Read the model definition and answer for the solid it produces. Units are mm, in the model's axes. A direction names the side the tool comes from. Give positions to 0.01 mm unless a question says otherwise; leave off trailing zeros. Write each loop counter-clockwise with the first axis right and the second up, starting at its lowest first coordinate (ties: lowest second). Pieces come first, ordered by that corner, then holes. Notation, with made-up numbers: (24.25, 14) - (76.25, 14) arc R27 ccw to (76.25, 34) - close; hole circle Ø9 at (-9, 58.5). An arc over 180 degrees is marked (long way). Use CSV: the item, a comma, the result in double quotes. Start each with the question number.
from build123d import *

# Parameters (mm, degrees)
F1_DEPTH = 50.8
F2_R     = 6.35
F3_R     = 1.016


# Not quite as in the source:
# - a fillet or chamfer that OpenCascade refuses, or shapes differently, is made with other operations: its cross-section is extruded or revolved along the edge and cut away or added


with BuildPart() as f1:
    # F0 (on Top) → F1 (new body)
    with BuildSketch(Plane.XY):
        with BuildLine():
            ThreePointArc((-2.6150272293, 15.9155984364), (-1.9815871124, 16.0068095983), (-1.3450272293, 16.07282))
            Line((-1.3450272293, 16.07282), (-1.3450272293, 21.15282))
            Line((-1.3450272293, 21.15282), (-2.6150272293, 21.15282))
            Line((-2.6150272293, 21.15282), (-2.6150272293, 15.9155984364))
        make_face()
        with BuildLine():
            Line((1.3450272293, 21.15282), (1.3450272293, 16.07282))
            ThreePointArc((1.3450272293, 16.07282), (1.9815871124, 16.0068095983), (2.6150272293, 15.9155984364))
            Line((2.6150272293, 15.9155984364), (2.6150272293, 21.15282))
            Line((2.6150272293, 21.15282), (1.3450272293, 21.15282))
        make_face()
        with BuildLine():
            ThreePointArc((0, 15.621), (11.0457150289, 11.0457150289), (15.621, 0))
            ThreePointArc((15.621, 0), (15.0887273325, -4.0430123035), (13.5281828325, -7.8105))
            Line((13.5281828325, -7.8105), (13.9681237376, -8.0645))
            ThreePointArc((13.9681237376, -8.0645), (14.2925051104, -7.4745527405), (14.5919840451, -6.8715822506))
            ThreePointArc((14.5919840451, -6.8715822506), (14.8530973018, -6.28730002), (15.090826177, -5.693119206))
            ThreePointArc((15.090826177, -5.693119206), (15.867333998, -2.8935018222), (16.129, 0))
            ThreePointArc((16.129, 0), (12.2947634215, 10.439513083), (2.6150272293, 15.9155984364))
            ThreePointArc((2.6150272293, 15.9155984364), (1.9815871124, 16.0068095983), (1.3450272293, 16.07282))
            ThreePointArc((1.3450272293, 16.07282), (0.6731, 16.1149488795), (0, 16.129))
            Line((0, 16.129), (0, 15.621))
        make_face()
        with BuildLine():
            ThreePointArc((15.090826177, -5.693119206), (14.8530973018, -6.28730002), (14.5919840451, -6.8715822506))
            Line((14.5919840451, -6.8715822506), (18.9913930963, -9.4115822506))
            Line((18.9913930963, -9.4115822506), (19.6263930963, -8.3117299878))
            Line((19.6263930963, -8.3117299878), (15.090826177, -5.693119206))
        make_face()
        with BuildLine():
            Line((17.646365867, -11.7412377494), (13.2469568158, -9.2012377494))
            ThreePointArc((13.2469568158, -9.2012377494), (12.8744329677, -9.7156377434), (12.4819459699, -10.2149726287))
            Line((12.4819459699, -10.2149726287), (16.8813550211, -12.7549726287))
            Line((16.8813550211, -12.7549726287), (17.646365867, -11.7412377494))
        make_face()
        with BuildLine():
            Line((13.9681237376, -8.0645), (13.5281828325, -7.8105))
            ThreePointArc((13.5281828325, -7.8105), (0, -15.621), (-13.5281828325, -7.8105))
            Line((-13.5281828325, -7.8105), (-13.9681237376, -8.0645))
            ThreePointArc((-13.9681237376, -8.0645), (-13.6194051104, -8.6403961391), (-13.2469568158, -9.2012377494))
            ThreePointArc((-13.2469568158, -9.2012377494), (-12.8744329677, -9.7156377434), (-12.4819459699, -10.2149726287))
            ThreePointArc((-12.4819459699, -10.2149726287), (0, -16.129), (12.4819459699, -10.2149726287))
            ThreePointArc((12.4819459699, -10.2149726287), (12.8744329677, -9.7156377434), (13.2469568158, -9.2012377494))
            ThreePointArc((13.2469568158, -9.2012377494), (13.6194051104, -8.6403961391), (13.9681237376, -8.0645))
        make_face()
        with BuildLine():
            ThreePointArc((-12.4819459699, -10.2149726287), (-12.8744329677, -9.7156377434), (-13.2469568158, -9.2012377494))
            Line((-13.2469568158, -9.2012377494), (-17.646365867, -11.7412377494))
            Line((-17.646365867, -11.7412377494), (-16.8813550211, -12.7549726287))
            Line((-16.8813550211, -12.7549726287), (-12.4819459699, -10.2149726287))
        make_face()
        with BuildLine():
            ThreePointArc((-13.5281828325, -7.8105), (-13.5281828325, 7.8105), (0, 15.621))
            Line((0, 15.621), (0, 16.129))
            ThreePointArc((0, 16.129), (-0.6731, 16.1149488795), (-1.3450272293, 16.07282))
            ThreePointArc((-1.3450272293, 16.07282), (-1.9815871124, 16.0068095983), (-2.6150272293, 15.9155984364))
            ThreePointArc((-2.6150272293, 15.9155984364), (-13.970548685, 8.0602984088), (-15.0873987804, -5.7021959842))
            ThreePointArc((-15.0873987804, -5.7021959842), (-14.8512055836, -6.2917671377), (-14.5919840451, -6.8715822506))
            ThreePointArc((-14.5919840451, -6.8715822506), (-14.2925051104, -7.4745527405), (-13.9681237376, -8.0645))
            Line((-13.9681237376, -8.0645), (-13.5281828325, -7.8105))
        make_face()
        with BuildLine():
            Line((-18.9913930963, -9.4115822506), (-14.5919840451, -6.8715822506))
            ThreePointArc((-14.5919840451, -6.8715822506), (-14.8512055836, -6.2917671377), (-15.0873987804, -5.7021959842))
            Line((-15.0873987804, -5.7021959842), (-19.4868078316, -8.2421959842))
            Line((-19.4868078316, -8.2421959842), (-18.9913930963, -9.4115822506))
        make_face()
    extrude(amount=F1_DEPTH)

    # F2
    f2_edges = [f1.edges().sort_by_distance(p)[0] for p in [
        (2.615027, 15.915598, 25.4),
        (15.090826, -5.693119, 25.4),
        (12.481946, -10.214973, 25.4),
        (-12.481946, -10.214973, 25.4),
        (-15.087399, -5.702196, 25.4),
        (-2.615027, 15.915598, 25.4),
    ]]
    fillet(f2_edges, radius=F2_R)

    # F3
    f3_edges = [f1.edges().sort_by_distance(p)[0] for p in [
        (1.345027, 21.15282, 25.4),
        (-1.345027, 21.15282, 25.4),
        (-18.991393, -9.411582, 25.4),
        (-17.646366, -11.741238, 25.4),
        (17.646366, -11.741238, 25.4),
        (18.991393, -9.411582, 25.4),
    ]]
    fillet(f3_edges, radius=F3_R)

    # F4: fillet of radius 1.016 on 1 edges, made by hand

    # F4_s1 → F4_t2 (revolve, cut)
    with BuildSketch(Plane.YZ):
        with BuildLine():
            ThreePointArc((15.621, 49.784), (15.9185795103, 50.5024204897), (16.637, 50.8))
            Line((16.637, 50.8), (15.621, 50.8))
            Line((15.621, 50.8), (15.621, 49.784))
        make_face()
    revolve(axis=Axis((0, 0, 50.8), (0, 0, -1)), mode=Mode.SUBTRACT)


solid = f1.part
(1) The part is cut by section A-A on y = 18.5. Write down the section's boundary in (x, z), plus the area to 3 significant figures.
(2) For a pull along X with two mould halves and no side action, classify faces 1 (the face through (-2, 18, 50.8)), 2 (the face through (-16.64, -5.364, 25.756)), 3 (the face through (12.965, -11.728, 25.756)) as pulls with the +X half, pulls with the -X half, needs draft (parallel to the pull), parting line crosses it, or undercut.
(3) Which of the six approach directions +Z, -Z, +X, -X, +Y, -Y give full straight-line access (tool end or side, diameter ignored) to faces 4 (the face through (16.327, -7.873, 25.044)), 5 (the face through (14.973, -10.198, 25.044)), 6 (the face through (1.345, 18, 25))?
(4) Consider probe 1 along X at (y, z) = (-7, 24); probe 2 along X at (y, z) = (0.5, 45); probe 3 along Y at (x, z) = (-4.5, 46.5). Determine where each line is inside the solid, lowest interval first.
(5) Given P1, Ø4, axis at y = -7.5, z = 25.5, coming from the -X side; P2, Ø0.6, axis at y = 21, z = 34.5, coming from the -X side (3 decimals); P3, Ø1, axis at y = 14.5, z = 36.5, coming from the -X side, each flat-ended and moving along its own axis, determine where each tip first touches the part or whether it passes through.
Reported:
1,outline,"(-2.98, 0) - (-1.35, 0) - (-1.35, 50.8) - (-2.98, 50.8) - close; (1.35, 0) - (2.98, 0) - (2.98, 50.8) - (1.35, 50.8) - close"
1,area,"166 mm²"
2,face 1,"needs draft"
2,face 2,"pulls with the -X half"
2,face 3,"undercut"
3,face 4,"+Z, -Z"
3,face 5,"+Z, -Z, +X"
3,face 6,"+Z, -Z, +Y"
4,probe 1,"-17.8 to -14.81, -14.53 to -13.96, 13.96 to 14.53, 14.81 to 17.81"
4,probe 2,"-16.12 to -15.61, 15.61 to 16.12"
4,probe 3,"-15.49 to -14.96, 14.96 to 16.1"
5,P1,"x = -19.49"
5,P2,"x = -2.615"
5,P3,"x = -8.01"
